The listing builds one solid part. Answer for the finished solid, in the listing's coordinates (mm). Face numbers are marked on the shaded views. A direction names the side the tool comes from. Give positions to 0.01 mm unless a question says otherwise; leave off trailing zeros. Loops run counter-clockwise (first coordinate to the right, second up) from the corner with the lowest first, then second, coordinate; pieces in that order, holes last. Notation, with made-up numbers: (11, 2.25) -> (43, 2.25) arc R13 cw to (43, 20.25) -> close; hole circle Ø6 at (62, 26.25). An arc over 180 degrees is marked (long way). One line per question, with ' | ' between items. Start each with the question number.
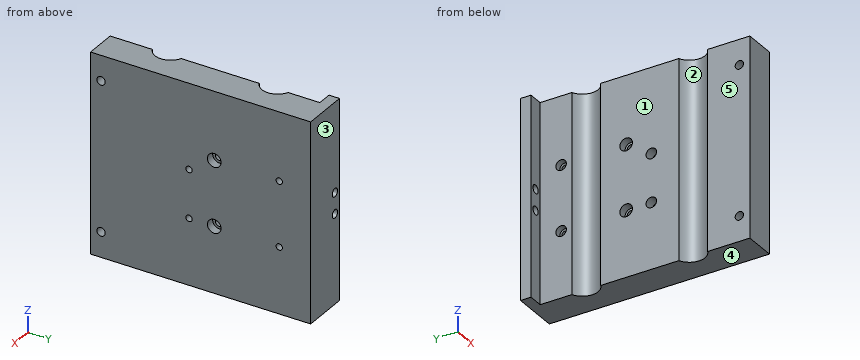
from build123d import *

# Parameters (mm, degrees)
BOSS_EXTRUDE1_DEPTH                = 95
SKETCH2_R                          = 2
CUT_EXTRUDE1_3DPRINTER4_DEPTH      = 139.744369255
ESQUISSE1_R                        = 1.5
ENL_V_MAT_EXTRU_1_3D_PRINTER_DEPTH = 140.67462189
ENL_V_MAT_EXTRU_2_DEPTH            = 139.744369255
ENL_V_MAT_EXTRU_2_DEPTH_BACK       = 3
ESQUISSE2_R                        = 2.5
ESQUISSE3_R                        = 3.25
ENL_V_MAT_EXTRU_3_DEPTH            = 4
ESQUISSE4_R                        = 2
ENL_V_MAT_EXTRU_4_DEPTH            = 140.67462189
ESQUISSE8_R                        = 7.5
ENL_V_MAT_EXTRU_9_DEPTH            = 139.744369255
ESQUISSE10_R                       = 2
ENL_V_MAT_EXTRU_10_DEPTH           = 139.744369255
ESQUISSE11_R                       = 2.5
ENL_V_MAT_EXTRU_11_DEPTH           = 5
ESQUISSE12_R                       = 3
ENL_V_MAT_EXTRU_12_DEPTH           = 4


with BuildPart() as part:
    # Sketch1 → Boss-Extrude1 (new body)
    with BuildSketch(Plane.XY):
        Polygon((0, 0), (0, -37.75), (0, -100), (15, -100), (15, 5), (-7, 5), (-7, 0), align=None)
    extrude(amount=BOSS_EXTRUDE1_DEPTH)

    # Sketch2 → Cut-Extrude1 3dprinter4 (cut, through all)
    with BuildSketch(Plane.ZY):
        with Locations(Location((62.5, -41, 0), (0, 0, 270))):
            Circle(SKETCH2_R)
        with Locations(Location((31.5, -41, 0), (0, 0, 270))):
            Circle(SKETCH2_R)
    extrude(amount=-CUT_EXTRUDE1_3DPRINTER4_DEPTH, mode=Mode.SUBTRACT)

    # Esquisse1 → Enlèv. mat.-Extru.1 3d printer (cut, through all)
    with BuildSketch(Plane(origin=(15, 0, 0), x_dir=(0, 0, -1), z_dir=(1, 0, 0))):
        with Locations(Location((-62.5, -10, 0), (0, 0, 90))):
            Circle(ESQUISSE1_R)
        with Locations(Location((-31.5, -10, 0), (0, 0, 90))):
            Circle(ESQUISSE1_R)
        with Locations(Location((-54.5, -53, 0), (0, 0, 90))):
            Circle(ESQUISSE1_R)
        with Locations(Location((-31.5, -53, 0), (0, 0, 90))):
            Circle(ESQUISSE1_R)
    extrude(amount=-ENL_V_MAT_EXTRU_1_3D_PRINTER_DEPTH, mode=Mode.SUBTRACT)

    # Esquisse2 → Enlèv. mat.-Extru.2 (cut, two sides: drawn at the far end of the back side and taken through both)
    with BuildSketch(Plane.ZY.offset(-ENL_V_MAT_EXTRU_2_DEPTH_BACK)):
        with Locations(Location((62.5, -10, 0), (0, 0, 90))):
            Circle(ESQUISSE2_R)
        with Locations(Location((31.5, -10, 0), (0, 0, 90))):
            Circle(ESQUISSE2_R)
    extrude(amount=ENL_V_MAT_EXTRU_2_DEPTH + ENL_V_MAT_EXTRU_2_DEPTH_BACK, mode=Mode.SUBTRACT)

    # Esquisse3 → Enlèv. mat.-Extru.3 (cut)
    with BuildSketch(Plane(origin=(15, 0, 0), x_dir=(0, 0, -1), z_dir=(1, 0, 0))):
        with Locations(Location((-31.5, -41, 0), (0, 0, 90))):
            Circle(ESQUISSE3_R)
        with Locations(Location((-62.5, -41, 0), (0, 0, 90))):
            Circle(ESQUISSE3_R)
    extrude(amount=-ENL_V_MAT_EXTRU_3_DEPTH, mode=Mode.SUBTRACT)

    # Esquisse4 → Enlèv. mat.-Extru.4 (cut, through all)
    with BuildSketch(Plane(origin=(15, 0, 0), x_dir=(0, 0, -1), z_dir=(1, 0, 0))):
        with Locations(Location((-83, -95, 0), (0, 0, 90))):
            Circle(ESQUISSE4_R)
        with Locations(Location((-12, -95, 0), (0, 0, 90))):
            Circle(ESQUISSE4_R)
    extrude(amount=-ENL_V_MAT_EXTRU_4_DEPTH, mode=Mode.SUBTRACT)

    # Esquisse8 → Enlèv. mat.-Extru.9 (cut, through all)
    with BuildSketch(Plane(origin=(0, 0, 0), x_dir=(-1, 0, 0), z_dir=(0, 0, -1))):
        with Locations((3, -22)):
            Circle(ESQUISSE8_R)
        with Locations((3, -73)):
            Circle(ESQUISSE8_R)
    extrude(amount=-ENL_V_MAT_EXTRU_9_DEPTH, mode=Mode.SUBTRACT)

    # Esquisse10 → Enlèv. mat.-Extru.10 (cut, through all)
    with BuildSketch(Plane.XZ):
        with Locations(Location((-3.5, 52.5, 0), (0, 0, 270))):
            Circle(ESQUISSE10_R)
        with Locations(Location((-3.5, 42.5, 0), (0, 0, 270))):
            Circle(ESQUISSE10_R)
    extrude(amount=-ENL_V_MAT_EXTRU_10_DEPTH, mode=Mode.SUBTRACT)

    # Esquisse11 → Enlèv. mat.-Extru.11 (cut)
    with BuildSketch(Plane.ZY):
        with Locations(Location((54.5, -53, 0), (0, 0, 270))):
            Circle(ESQUISSE11_R)
        with Locations(Location((31.5, -53, 0), (0, 0, 270))):
            Circle(ESQUISSE11_R)
    extrude(amount=-ENL_V_MAT_EXTRU_11_DEPTH, mode=Mode.SUBTRACT)

    # Esquisse12 → Enlèv. mat.-Extru.12 (cut)
    with BuildSketch(Plane.ZY):
        with Locations(Location((62.5, -41, 0), (0, 0, 270))):
            Circle(ESQUISSE12_R)
        with Locations(Location((31.5, -41, 0), (0, 0, 270))):
            Circle(ESQUISSE12_R)
    extrude(amount=-ENL_V_MAT_EXTRU_12_DEPTH, mode=Mode.SUBTRACT)


solid = part.part
1. Each of these flat-tipped pins is pushed along its axis until it touches: pin 1 Ø6.5 at (y, z) = (-41.5, 62) entering from -X; pin 2 Ø3.5 at (x, z) = (-5, 68.5) entering from -Y; pin 3 Ø3.5 at (y, z) = (-95, 12) entering from +X; pin 4 Ø4.5 at (y, z) = (-53, 54.5) entering from -X. Where does it stop, or does it pass through?
2. Determine the mould class of the marked faces 1, 2 and 3 for opening direction Y: released by +Y, released by -Y, zero draft, split by the parting line, or undercut.
3. Straight lines are drawn through the part: L1, parallel to Z at x = 6.5, y = -41; L2, parallel to Z at x = 2.05, y = -53; L3, parallel to Y at x = 0.5, z = 61. For each, find the intervals that lie inside material, in ascending order.
4. The part is cut by section C-C (z = 12). Write down the section's boundary in (x, y), plus the area to 3 significant figures.
5. For the marked faces 4 and 5, determine the directions among +Z, -Z, +X, -X, +Y, -Y from which every point of the face is accessible in a straight line to the end or side of a thin tool.
6. The part is cut by section A-A (y = -41). Write down the section's boundary in (x, z).
7. The part is cut by section B-B (x = 1.25). Count the separate pieces of the cut face and the enclosed holes in it, plus the area to 3 significant figures.
Check sheet entries:
1) pin 1: stops at x = 0 | pin 2: stops at y = 0 | pin 3: passes through | pin 4: stops at x = 5
2) face 1: zero draft | face 2: undercut | face 3: released by +Y
3) L1: z = 0 to 29.5, 33.5 to 60.5, 64.5 to 95 | L2: z = 0 to 29, 34 to 52, 57 to 95 | L3: y = -100 to -79.63, -66.37 to -43.6, -38.4 to -28.63, -15.37 to -12, -8 to 5
4) outline: (-7, 0) -> (0, 0) -> (0, -15.13) arc R7.5 cw to (0, -28.87) -> (0, -66.13) arc R7.5 cw to (0, -79.87) -> (0, -93) -> (15, -93) -> (15, 5) -> (-7, 5) -> close; (0, -100) -> (15, -100) -> (15, -97) -> (0, -97) -> close | area: 1,460 mm^2
5) face 4: -Z, +X, -X, +Y, -Y | face 5: +Z, -Z, -X, -Y
6) outline: (0, 0) -> (15, 0) -> (15, 28.25) -> (11, 28.25) -> (11, 29.5) -> (4, 29.5) -> (4, 28.5) -> (0, 28.5) -> close; (0, 34.5) -> (4, 34.5) -> (4, 33.5) -> (11, 33.5) -> (11, 34.75) -> (15, 34.75) -> (15, 59.25) -> (11, 59.25) -> (11, 60.5) -> (4, 60.5) -> (4, 59.5) -> (0, 59.5) -> close; (0, 65.5) -> (4, 65.5) -> (4, 64.5) -> (11, 64.5) -> (11, 65.75) -> (15, 65.75) -> (15, 95) -> (0, 95) -> close
7) separate pieces: 3 | enclosed holes: 8 | area: 7,470 mm^2
